The figure shows three views and two pictorial views of one solid part (mm, origin at its lowest corner). Answer the questions. Coordinates: 2 decimals unless noted, no trailing zeros. Loops run counter-clockwise (first coordinate to the right, second up) from the corner with the lowest first, then second, coordinate; pieces in that order, holes last.
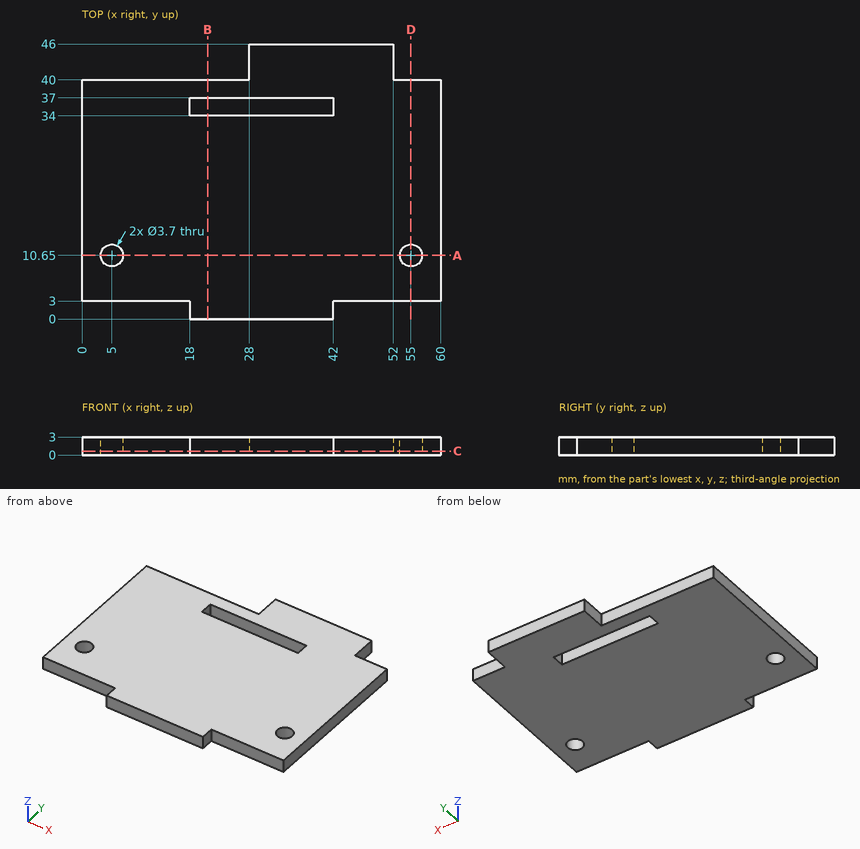
Q1. A cutting plane is placed at B-B (x = 21). Give the vertices of the cut face in (y, z).
Findings below:
outline: (0, 0) - (34, 0) - (34, 3) - (0, 3) - close; (37, 0) - (40, 0) - (40, 3) - (37, 3) - close
Q2. Straight lines are drawn through the part: probe 1 along X at (y, z) = (10.5, 1.7); probe 2 along Y at (x, z) = (20, 0.5); probe 3 along Y at (x, z) = (55, 0.9). For each, find the intervals that lie inside material, in ascending order.
Findings below:
probe 1: x = 0 to 3.16, 6.84 to 53.16, 56.84 to 60
probe 2: y = 0 to 34, 37 to 40
probe 3: y = 3 to 8.8, 12.5 to 40
Q3. A cutting plane is placed at D-D (x = 55). Give the vertices of the cut face in (y, z), then the cut area to 3 significant figures.
Findings below:
outline: (3, 0) - (8.8, 0) - (8.8, 3) - (3, 3) - close; (12.5, 0) - (40, 0) - (40, 3) - (12.5, 3) - close
area: 99.9 mm2
Q4. A cutting plane is placed at C-C (z = 0.65). Give the vertices of the cut face in (x, y), then the cut area to 3 significant figures.
Findings below:
outline: (0, 3) - (18, 3) - (18, 0) - (42, 0) - (42, 3) - (60, 3) - (60, 40) - (52, 40) - (52, 46) - (28, 46) - (28, 40) - (0, 40) - close; hole circle Ø3.7 at (5, 10.65); hole (18, 34) - (42, 34) - (42, 37) - (18, 37) - close; hole circle Ø3.7 at (55, 10.65)
area: 2,340 mm2
Q5. A cutting plane is placed at A-A (y = 10.65). Give the vertices of the cut face in (x, z).
Findings below:
outline: (0, 0) - (3.15, 0) - (3.15, 3) - (0, 3) - close; (6.85, 0) - (53.15, 0) - (53.15, 3) - (6.85, 3) - close; (56.85, 0) - (60, 0) - (60, 3) - (56.85, 3) - close
Q6. Flat-ended cylindrical pins translate along their axes: pin 1 Ø0.9 at (x, z) = (7.5, 1.5) entering from -Y; pin 2 Ø0.9 at (y, z) = (1.5, 1.5) entering from +X; pin 3 Ø1.5 at (y, z) = (42, 1.5) entering from +X. Find the tip coordinate at first contact, or state that the pin passes through.
Findings below:
pin 1: stops at y = 3
pin 2: stops at x = 42
pin 3: stops at x = 52
